The model under review builds one solid part; all positions refer to its coordinate system, in mm. Face numbers are marked on the shaded views. Give positions to 0.01 mm unless a question says otherwise; leave off trailing zeros. Write each loop counter-clockwise with the first axis right and the second up, starting at its lowest first coordinate (ties: lowest second). Pieces come first, ordered by that corner, then holes. Notation, with made-up numbers: (37.25, 42) -> (65.25, 42) arc R7 ccw to (65.25, 53) -> close; hole circle Ø1 at (59, 42). An arc over 180 degrees is marked (long way). Use CSV: the item, a comma, the result in double quotes.
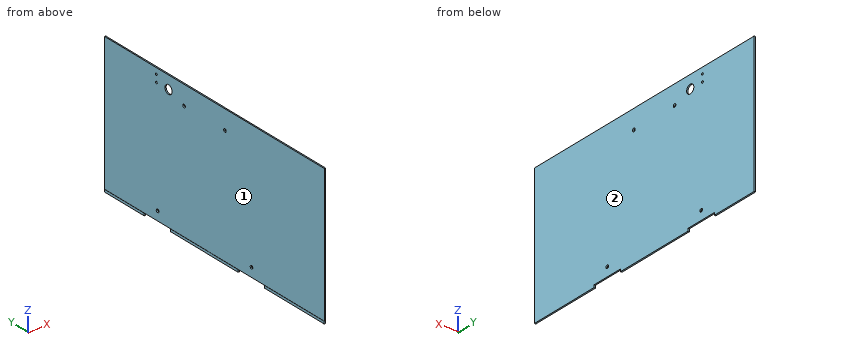
Autodesk Inventor part; units mm, degrees
ref_plane "作業平面1" through (0, 75.6523, 179.1954) normal (0, 1, 0) x (1, 0, 0)
ref_plane "YZ Plane" through (0, 0, 0) normal (1, 0, 0) x (0, 1, 0)
ref_plane "XZ Plane" through (0, 0, 0) normal (0, 1, 0) x (-1, 0, 0)
sketch "スケッチ1" plane through (0, 0, 0) normal (1, 0, 0) x (0, 1, 0)
  line L0 (125.6523, 179.1954) -> (-474.3477, 179.1954)
  line L1 (-474.3477, 179.1954) -> (-474.3477, -102.8046)
  line L2 (-474.3477, -102.8046) -> (125.6523, -102.8046)
  line L3 (125.6523, -102.8046) -> (125.6523, 179.1954)
  dimension "d0" = 600
  dimension "d1" = 282
extrude "押し出し1" add sketch "スケッチ1" along normal blind 2.6
sketch "スケッチ4" plane through (2.6, 0, 0) normal (1, 0, 0) x (0, 0, -1)
  line L0 (102.8046, 125.6523) -> (-179.1954, 125.6523)
  line L1 (-179.1954, 125.6523) -> (-179.1954, -474.3477)
  point P0 (0, 0)
  point P1 (-139.1954, -225.3477)
  point P2 (-139.1954, -123.3477)
  dimension "d19" = 102
  dimension "d20" = 249
  dimension "d21" = 40
  dimension "d22" = 40
hole "穴2" at (2.6, -225.3477, 139.1954) at (2.6, -123.3477, 139.1954) direction (-1, 0, 0) diameter 6.6 end through all
sketch "スケッチ5" plane through (2.6, 0, 0) normal (1, 0, 0) x (0, 0, -1)
  line L0 (-179.1954, 125.6523) -> (-179.1954, -474.3477)
  line L1 (102.8046, 125.6523) -> (-179.1954, 125.6523)
  point P0 (-152.1954, -84.3477)
  dimension "d30" = 27
  dimension "d31" = 210
hole "穴3" at (2.6, -84.3477, 152.1954) direction (-1, 0, 0) diameter 18 end through all
sketch "スケッチ6" plane through (2.6, 0, 0) normal (1, 0, 0) x (0, 0, -1)
  line L0 (-179.1954, 125.6523) -> (-179.1954, -474.3477)
  circle A0 centre (-152.1954, -84.3477) radius 9
  point P0 (0, 0)
  point P1 (-166.6954, -53.9477)
  point P2 (-151.6954, -53.9477)
  dimension "d39" = 12.5
  dimension "d40" = 27.5
  dimension "d41" = 30.4
  dimension "d42" = 30.4
hole "穴4" at (2.6, -53.9477, 166.6954) at (2.6, -53.9477, 151.6954) direction (-1, 0, 0) diameter 4.5 end through all
sketch "スケッチ7" plane through (2.6, 0, 0) normal (1, 0, 0) x (0, 0, -1)
  line L0 (102.8046, 125.6523) -> (-179.1954, 125.6523)
  line L1 (102.8046, -474.3477) -> (102.8046, 125.6523)
  line L2 (-179.1954, -474.3477) -> (102.8046, -474.3477)
  point P0 (0, 0)
  point P1 (84.0046, -56.9477)
  point P2 (84.0046, -291.9477)
  dimension "d50" = 182.6
  dimension "d51" = 18.8
  dimension "d52" = 18.8
  dimension "d53" = 182.4
hole "穴5" at (2.6, -56.9477, -84.0046) at (2.6, -291.9477, -84.0046) direction (-1, 0, 0) diameter 6.7 end through all
sketch "スケッチ8" plane through (2.6, 0, 0) normal (1, 0, 0) x (0, 0, -1)
  line L0 (102.8046, -474.3477) -> (102.8046, 125.6523)
  line L1 (102.8046, 125.6523) -> (107.8046, 125.6523)
  line L2 (117.7603, -23.9477) -> (102.8046, -23.9477)
  line L3 (102.8046, -89.9477) -> (117.7603, -89.9477)
  line L4 (107.8046, 125.6523) -> (107.8046, -474.3477)
  line L5 (107.8046, -474.3477) -> (102.8046, -474.3477)
  line L6 (102.8046, -258.9477) -> (107.8046, -258.9477)
  line L7 (102.8046, -324.9477) -> (107.8046, -324.9477)
  circle A0 centre (84.0046, -56.9477) radius 3.35
  circle A1 centre (84.0046, -291.9477) radius 3.35
  point P0 (0, 0)
  point P1 (107.8046, -23.9477)
  point P2 (107.8046, -89.9477)
  dimension "d61" = 5
  dimension "d62" = 33
  dimension "d63" = 33
  dimension "d64" = 33
  dimension "d65" = 33
extrude "押し出し3" add sketch "スケッチ8" against normal blind 3 contours L0 L7 L4 L5 | L0 L3 L4 L6 | L0 L1 L4 L2
sketch "スケッチ9" plane through (2.6, 0, 0) normal (1, 0, 0) x (0, 0, -1)
  ellipse E0 centre (-2.4593, 110.6523) end of major axis (-2.4593, 125.1521) minor radius 14.4996 (5.606, 98.6026) -> (5.606, 122.702) ccw
  line L0 (4.4935, 123.5363) -> (-99.9579, 123.5363)
  line L1 (-99.9579, 97.7683) -> (4.4935, 97.7683)
  ellipse E1 centre (-67.383, 110.6523) end of major axis (-67.383, 123.067) minor radius 12.4145 (-70.683, 122.6204) -> (-70.683, 98.6842) ccw
  line L2 (-70.683, 122.6204) -> (-70.683, 125.6523)
  line L3 (102.8046, 125.6523) -> (-179.1954, 125.6523)
  line L4 (5.7266, 122.6204) -> (5.7266, 125.6523)
  line L5 (5.7266, 125.6523) -> (-70.683, 125.6523)
  line L6 (6.1243, 98.9661) -> (4.4935, 97.7683)
  line L7 (-70.683, 98.6842) -> (-66.6998, 97.7683)
  point P0 (0, 0)
extrude "押し出し4" cut sketch "スケッチ9" against normal blind 3
ref_plane "作業平面1" through (0, 75.6523, 179.1954) normal (0, 1, 0) x (1, 0, 0)
split "分割1" plane through (0, 75.6523, 179.1954) removes the side toward (0, 1, 0)
properties part number "lc_box_side" material "ポリカーボネート、クリア"
Q1. Insertion check: pin 1 (4 mm diameter, centred on y = -337.5, z = 76.5, fed in from -X); pin 2 (0.8 mm diameter, centred on x = 2, y = -288.5, fed in from -Z). Each pin has a flat end and moves straight along its axis. Give the tip position at first contact, or say it passes through.
Derived:
pin 1,"stops at x = 0"
pin 2,"stops at z = -102.8"
Q2. To check wall thickness, follow probe 1 along X at (y, z) = (-39, 54.5); probe 2 along Z at (x, y) = (1.65, -298); probe 3 along Y at (x, z) = (0.05, 144.5). State the ranges of each line that lie inside material, in increasing order.
Derived:
probe 1,"x = 0 to 2.6"
probe 2,"z = -102.8 to 179.2"
probe 3,"y = -474.35 to -89.01, -79.68 to 75.65"
Q3. The part is to be moulded in two halves that separate along X. For the marked faces 1 and 2, say which applies: pulls with the +X half, pulls with the -X half, needs draft (parallel to the pull), parting line crosses it, or undercut.
Derived:
face 1,"pulls with the -X half"
face 2,"pulls with the +X half"
Q4. Consider section A-A (y = -345.5). Write out the cut boundary in (x, z).
Derived:
outline,"(-0.4, -107.8) -> (2.6, -107.8) -> (2.6, 179.2) -> (0, 179.2) -> (0, -102.8) -> (-0.4, -102.8) -> close"
Q5. Consider section B-B (z = 39). Write out the cut boundary in (x, y), then the cut area to 3 significant figures.
Derived:
outline,"(0, -474.35) -> (2.6, -474.35) -> (2.6, 75.65) -> (0, 75.65) -> close"
area,"1,430 mm2"
